Could you check a few things on this model? Use its own coordinates, in mm. Round coordinates to 2 decimals unless told otherwise and drop trailing zeros. Order: outer loops, then holes, each group sorted by start corner. A loop starts at its lowest first (then second) coordinate and runs counter-clockwise, first axis right, second up. Notation, with made-up numbers: M -5.5,-34 L 49.5,-34 A22 ccw 49.5,-18 Z; hole C 41,86.5 d9. An arc over 180 degrees is marked long. Write each question's results on one line, items separated by ' | '. Start each with the question number.
1. Suppose I cut it at A-A on x = -47. Write out the boundary of the cut face in (y, z).
2. Please list where these lines run through material, in increasing order: L1, parallel to X at y = 2.3, z = 55; L2, parallel to X at y = 1.6, z = -74; L3, parallel to Z at x = -67.5, y = 1.25.
3. I'm going to push a flat-ended pin straight in: pin 1 (2.5 mm diameter, centred on x = -33.5, z = -1.85, fed in from -Y). Where does the tip first touch, or does it pass through?
from build123d import *

# Parameters (mm, degrees)
SKETCH_1_R      = 1.6
SKETCH_1_R_2    = 1.7
SKETCH_1_W      = 3
SKETCH_1_H      = 7
SKETCH_1_W_2    = 7
SKETCH_1_H_2    = 3
EXTRUDE_2_DEPTH = 3


with BuildPart() as part:
    # 草图1 → 凸台-拉伸2 (new body)
    with BuildSketch(Plane(origin=(0, 0, 0), x_dir=(1, 0, 0), z_dir=(0, 1, 0))):
        with BuildLine():
            Line((67.5, 100), (-67.5, 100))
            ThreePointArc((-67.5, 100), (-71.035533906, 98.535533906), (-72.5, 95))
            Line((-72.5, 95), (-72.5, 43.7))
            Line((-72.5, 43.7), (-44.5, 43.7))
            Line((-44.5, 43.7), (-44.5, -21.3))
            Line((-44.5, -21.3), (-72.5, -21.3))
            Line((-72.5, -21.3), (-72.5, -95))
            ThreePointArc((-72.5, -95), (-71.035533906, -98.535533906), (-67.5, -100))
            Line((-67.5, -100), (67.5, -100))
            ThreePointArc((67.5, -100), (71.035533906, -98.535533906), (72.5, -95))
            Line((72.5, -95), (72.5, -21.3))
            Line((72.5, -21.3), (44.5, -21.3))
            Line((44.5, -21.3), (44.5, 43.7))
            Line((44.5, 43.7), (72.5, 43.7))
            Line((72.5, 43.7), (72.5, 95))
            ThreePointArc((72.5, 95), (71.035533906, 98.535533906), (67.5, 100))
        make_face()
        with Locations(Location((-67.5, -95, 0), (0, 0, 270))):
            Circle(SKETCH_1_R, mode=Mode.SUBTRACT)
        with Locations(Location((-19.5, -80, 0), (0, 0, 270))):
            Circle(SKETCH_1_R_2, mode=Mode.SUBTRACT)
        with Locations((-34, -51.69160916)):
            Rectangle(SKETCH_1_W, SKETCH_1_H, mode=Mode.SUBTRACT)
        with Locations(Location((-22, -10.8, 0), (0, 0, 270))):
            Circle(SKETCH_1_R_2, mode=Mode.SUBTRACT)
        with Locations((0, -79.69160916)):
            Rectangle(SKETCH_1_W_2, SKETCH_1_H_2, mode=Mode.SUBTRACT)
        with Locations(Location((19.5, -80, 0), (0, 0, 270))):
            Circle(SKETCH_1_R_2, mode=Mode.SUBTRACT)
        with Locations((34, -51.69160916)):
            Rectangle(SKETCH_1_W, SKETCH_1_H, mode=Mode.SUBTRACT)
        with Locations(Location((67.5, -95, 0), (0, 0, 270))):
            Circle(SKETCH_1_R, mode=Mode.SUBTRACT)
        with Locations(Location((33.5, -37.45, 0), (0, 0, 270))):
            Circle(SKETCH_1_R, mode=Mode.SUBTRACT)
        with Locations((0, -23.69160916)):
            Rectangle(SKETCH_1_W_2, SKETCH_1_H_2, mode=Mode.SUBTRACT)
        with Locations(Location((25.5, -23.45, 0), (0, 0, 270))):
            Circle(SKETCH_1_R, mode=Mode.SUBTRACT)
        with Locations(Location((22, -10.8, 0), (0, 0, 270))):
            Circle(SKETCH_1_R_2, mode=Mode.SUBTRACT)
        with Locations(Location((-33.5, 1.85, 0), (0, 0, 270))):
            Circle(SKETCH_1_R, mode=Mode.SUBTRACT)
        with Locations(Location((-25.5, 15.85, 0), (0, 0, 270))):
            Circle(SKETCH_1_R, mode=Mode.SUBTRACT)
        with Locations(Location((-22, 33.2, 0), (0, 0, 270))):
            Circle(SKETCH_1_R_2, mode=Mode.SUBTRACT)
        with Locations(Location((-25.5, 45.85, 0), (0, 0, 270))):
            Circle(SKETCH_1_R, mode=Mode.SUBTRACT)
        with Locations(Location((-67.5, 95, 0), (0, 0, 270))):
            Circle(SKETCH_1_R, mode=Mode.SUBTRACT)
        with Locations(Location((-33.5, 59.85, 0), (0, 0, 270))):
            Circle(SKETCH_1_R, mode=Mode.SUBTRACT)
        with Locations(Location((-33.15, 74, 0), (0, 0, 270))):
            Circle(SKETCH_1_R_2, mode=Mode.SUBTRACT)
        with BuildLine():
            ThreePointArc((-10, 18.30839084), (-9.121320344, 20.429711183), (-7, 21.30839084))
            Line((-7, 21.30839084), (7, 21.30839084))
            ThreePointArc((7, 21.30839084), (9.121320344, 20.429711183), (10, 18.30839084))
            Line((10, 18.30839084), (10, 4.30839084))
            ThreePointArc((10, 4.30839084), (9.121320344, 2.187070496), (7, 1.30839084))
            Line((7, 1.30839084), (-7, 1.30839084))
            ThreePointArc((-7, 1.30839084), (-9.121320344, 2.187070496), (-10, 4.30839084))
            Line((-10, 4.30839084), (-10, 18.30839084))
        make_face(mode=Mode.SUBTRACT)
        with Locations(Location((25.5, 6.55, 0), (0, 0, 270))):
            Circle(SKETCH_1_R, mode=Mode.SUBTRACT)
        with Locations(Location((33.5, 20.55, 0), (0, 0, 270))):
            Circle(SKETCH_1_R, mode=Mode.SUBTRACT)
        with Locations(Location((22, 33.30839084, 0), (0, 0, 270))):
            Circle(SKETCH_1_R_2, mode=Mode.SUBTRACT)
        with Locations(Location((0, 74, 0), (0, 0, 270))):
            Circle(SKETCH_1_R_2, mode=Mode.SUBTRACT)
        with Locations(Location((33.15, 74, 0), (0, 0, 270))):
            Circle(SKETCH_1_R_2, mode=Mode.SUBTRACT)
        with Locations(Location((67.5, 95, 0), (0, 0, 270))):
            Circle(SKETCH_1_R, mode=Mode.SUBTRACT)
    extrude(amount=EXTRUDE_2_DEPTH)


solid = part.part
Filled sheet:
1) outline: M 0,-100 L 3,-100 L 3,-43.7 L 0,-43.7 Z; M 0,21.3 L 3,21.3 L 3,100 L 0,100 Z
2) L1: x = -72.5 to -35.5, -32.5 to 32.5, 35.5 to 72.5 | L2: x = -72.5 to -34.85, -31.45 to -1.7, 1.7 to 31.45, 34.85 to 72.5 | L3: z = -100 to -96.6, -93.4 to -43.7, 21.3 to 93.4, 96.6 to 100
3) pin 1: passes through
